Geometry: see drawing. Coordinates: mm, zero at the bounding-box minimum. A direction names the side the tool comes from. Round coordinates to 2 decimals unless told otherwise and drop trailing zeros. Loops run counter-clockwise (first coordinate to the right, second up) from the corner with the lowest first, then second, coordinate; pieces in that order, holes last. Notation, with made-up numbers: (-19, 72) - (32, 72) arc R28 cw to (32, 94) - close; hole circle Ø5 at (4, 65.5). An arc over 180 degrees is marked (long way). Answer in a Markdown table with one row per item. Add a question column.
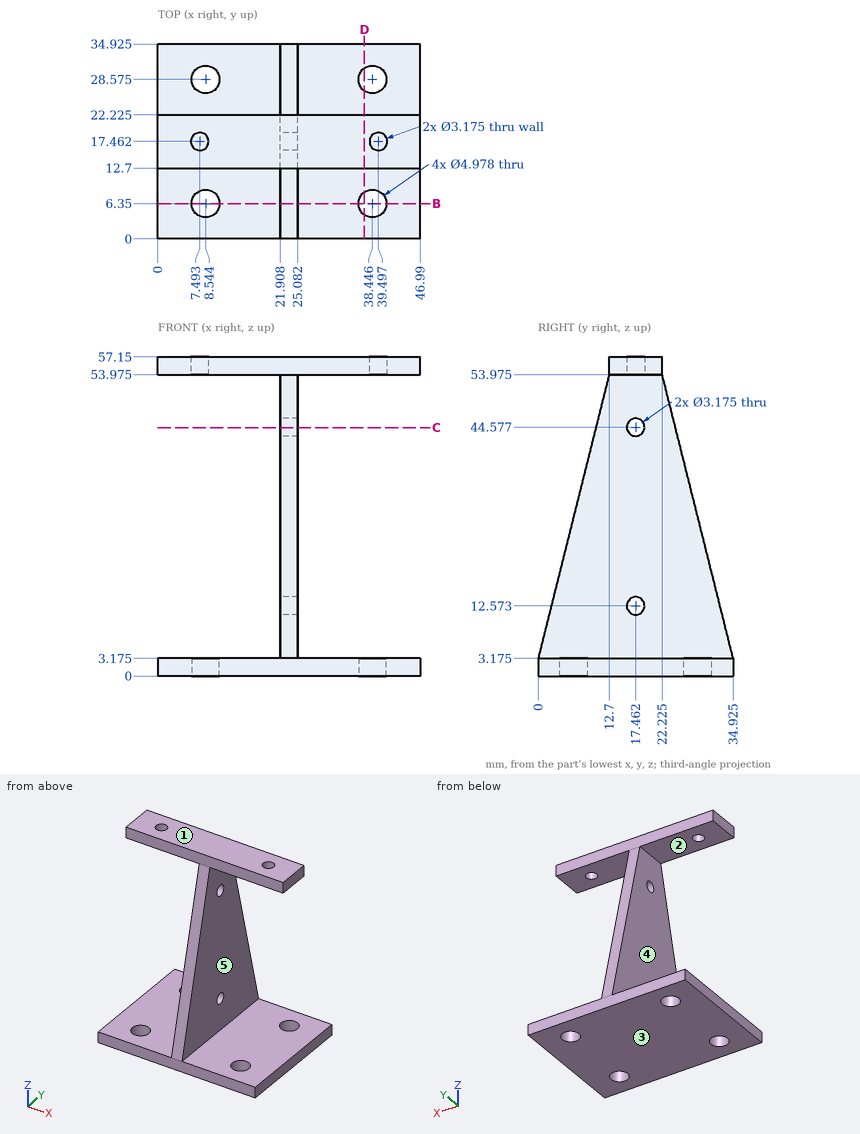
1) Section C-C, the plane z = 44.5. Return the cut outline in (x, y).
2) Material intervals for line 1 along X through (y, z) = (22.5, 40); line 2 along Z through (x, y) = (42.5, 10) (1 decimal); line 3 along Y through (x, z) = (23, 47) (1 decimal), sorted ascending. Write a range as from..to.
3) Section B-B, the plane y = 6.35. Return the cut outline in (x, z) (1 decimal).
4) Pull-direction query (Z, two-part tool) for the marked faces 1, 2 and 3; classes: pulls with the +Z half, pulls with the -Z half, needs draft (parallel to the pull), parting line crosses it, or undercut.
5) Contact query for flat-ended pins moving along their axis: pin 1 Ø8 at (x, y) = (38.45, 28.58) entering from +Z (1 decimal); pin 2 Ø10.5 at (y, z) = (11.5, 22) entering from +X; pin 3 Ø5 at (x, y) = (7.49, 17.46) entering from +Z; pin 4 Ø2 at (x, z) = (20.5, 17) entering from -Y. Output: stop coordinate, or through.
6) Section D-D, the plane x = 37. Give the number of separate pieces and of enclosed holes in the cut face, and give its area (3 significant figures).
7) Reachability of the marked faces 4 and 5 from +Z, -Z, +X, -X, +Y, -Y: full face, straight path, thin tool, end or side. Return the list, or none.
Evaluation:
| question | item | result |
|---|---|---|
| 1 | outline | (21.91, 10.33) - (25.08, 10.33) - (25.08, 15.88) - (21.91, 15.88) - close; (21.91, 19.05) - (25.08, 19.05) - (25.08, 24.59) - (21.91, 24.59) - close |
| 2 | line 1 | x = 21.91..25.08 |
| 2 | line 2 | z = 0..3.2 |
| 2 | line 3 | y = 11..24 |
| 3 | outline | (0, 0) - (6.1, 0) - (6.1, 3.2) - (0, 3.2) - close; (11, 0) - (36, 0) - (36, 3.2) - (25.1, 3.2) - (25.1, 28.6) - (21.9, 28.6) - (21.9, 3.2) - (11, 3.2) - close; (40.9, 0) - (47, 0) - (47, 3.2) - (40.9, 3.2) - close |
| 4 | face 1 | pulls with the +Z half |
| 4 | face 2 | undercut |
| 4 | face 3 | pulls with the -Z half |
| 5 | pin 1 | stops at z = 3.2 |
| 5 | pin 2 | stops at x = 25.08 |
| 5 | pin 3 | stops at z = 57.15 |
| 5 | pin 4 | passes through |
| 6 | separate pieces | 4 |
| 6 | enclosed holes | 0 |
| 6 | area | 115 mm² |
| 7 | face 4 | -X, +Y, -Y |
| 7 | face 5 | +X, +Y, -Y |
